```python
from build123d import *

# Parameters (mm, degrees)
F1_DEPTH = 4.5


with BuildPart() as f1:
    # F0 (on Top) → F1 (new body)
    with BuildSketch(Plane.XY):
        with BuildLine():
            Line((-6.747654, 8.625), (3.625, 8.625))
            ThreePointArc((3.625, 8.625), (7.160534, 7.160534), (8.625, 3.625))
            Line((8.625, 3.625), (8.625, -3.625))
            ThreePointArc((8.625, -3.625), (7.160534, -7.160534), (3.625, -8.625))
            Line((3.625, -8.625), (-6.747654, -8.625))
            ThreePointArc((-6.747654, -8.625), (-8.505197, -8.944076), (-10.038423, -9.860582))
            Line((-10.038423, -9.860582), (-12.049675, -11.618772))
            ThreePointArc((-12.049675, -11.618772), (1.752407, -16.64691), (14.204929, -8.854971))
            ThreePointArc((14.204929, -8.854971), (16.021618, -7.128207), (18.44802, -6.5))
            Line((18.44802, -6.5), (43.625, -6.5))
            ThreePointArc((43.625, -6.5), (47.160534, -5.035534), (48.625, -1.5))
            Line((48.625, -1.5), (48.625, 1.5))
            ThreePointArc((48.625, 1.5), (47.160534, 5.035534), (43.625, 6.5))
            Line((43.625, 6.5), (18.44802, 6.5))
            ThreePointArc((18.44802, 6.5), (16.021618, 7.128207), (14.204929, 8.854971))
            ThreePointArc((14.204929, 8.854971), (1.752407, 16.64691), (-12.049675, 11.618772))
            Line((-12.049675, 11.618772), (-10.038423, 9.860582))
            ThreePointArc((-10.038423, 9.860582), (-8.505197, 8.944076), (-6.747654, 8.625))
        make_face()
    extrude(amount=F1_DEPTH)


solid = f1.part
```
Here's how the part is built. I have some questions about the finished solid (model axes, mm). A direction names the side the tool comes from. Round coordinates to 2 decimals unless told otherwise and drop trailing zeros. Order: outer loops, then holes, each group sorted by start corner. A loop starts at its lowest first (then second) coordinate and runs counter-clockwise, first axis right, second up. Notation, with made-up numbers: M -23.75,-32 L 23.25,-32 A21 ccw 23.25,-7 Z; hole C 75.5,23 d2. An arc over 180 degrees is marked long. Use CSV: the item, a comma, the result in double quotes.
1) I want a section at A-A (x = 0). List the corners of the cut face in (y, z) for me (3 decimals), then the cut area to 3 significant figures.
Taken from the geometry:
outline,"M -16.739,0 L -8.625,0 L -8.625,4.5 L -16.739,4.5 Z; M 8.625,0 L 16.739,0 L 16.739,4.5 L 8.625,4.5 Z"
area,"73.0 mm^2"
2) If we mould it in two halves opening along Y, with no side actions, what happens to faces 1 (the cylindrical face through (47.121, -5.074, 2.218)), 2 (the flat face through (-1, -8.625, 2)), 3 (the cylindrical face through (47.199, 4.996, 2.218))? For each: pulls with the +Y half, pulls with the -Y half, needs draft (parallel to the pull), parting line crosses it, or undercut.
Taken from the geometry:
face 1,"pulls with the -Y half"
face 2,"undercut"
face 3,"pulls with the +Y half"
3) I want a section at B-B (z = 2.2). List the corners of the cut face in (x, y) for me (3 decimals), then the cut area to 3 significant figures.
Taken from the geometry:
outline,"M -12.05,-11.619 A16.739 ccw 14.205,-8.855 A5 cw 18.448,-6.5 L 43.625,-6.5 A5 ccw 48.625,-1.5 L 48.625,1.5 A5 ccw 43.625,6.5 L 18.448,6.5 A5 cw 14.205,8.855 A16.739 ccw -12.05,11.619 L -10.038,9.861 A5 ccw -6.748,8.625 L 3.625,8.625 A5 cw 8.625,3.625 L 8.625,-3.625 A5 cw 3.625,-8.625 L -6.748,-8.625 A5 ccw -10.038,-9.861 Z"
area,"861 mm^2"
4) I'm going to push flat-ended pins straight in: P1, Ø2, axis at y = -1.5, z = 3.5, coming from the -X side (3 decimals); P2, Ø2, axis at x = 37.5, z = 1.5, coming from the +Y side; P3, Ø2, axis at x = 16.5, z = 1, coming from the +Y side. Where does each tip first touch, or does it pass through?
Taken from the geometry:
P1,"x = 8.625"
P2,"y = 6.5"
P3,"y = 7.46"
5) I need wall thicknesses on line 1 along X through (y, z) = (1, 3.6) (3 decimals); line 2 along Y through (x, z) = (31, 1.7); line 3 along Y through (x, z) = (3, 2.4) (3 decimals). Which ranges of each line are inside material? Lowest first, please. Write a range as [from, to].
Taken from the geometry:
line 1,"[8.625, 48.625]"
line 2,"[-6.5, 6.5]"
line 3,"[-16.468, -8.625], [8.625, 16.468]"
6) I want a section at D-D (x = 30). List the corners of the cut face in (y, z) for me, then the cut area to 3 significant figures.
Taken from the geometry:
outline,"M -6.5,0 L 6.5,0 L 6.5,4.5 L -6.5,4.5 Z"
area,"58.5 mm^2"
7) I want a section at C-C (y = -8). List the corners of the cut face in (x, z) for me.
Taken from the geometry:
outline,"M 6.05,0 L 14.88,0 L 14.88,4.5 L 6.05,4.5 Z"
8) On a 3-axis mill with a long thin cutter (end or side, diameter ignored), from which of +Z, -Z, +X, -X, +Y, -Y can I reach the whole of each face in a straight line? I mean faces 4 (the flat face through (31, 6.5, 2)), 5 (the flat face through (18, 0, 0)), 6 (the cylindrical face through (7.12, 7.2, 2.22)), 7 (the flat face through (31, -6.5, 2)). Say none if no direction works.
Taken from the geometry:
face 4,"+Z, -Z, +X, +Y"
face 5,"-Z, +X, -X, +Y, -Y"
face 6,"+Z, -Z, -X"
face 7,"+Z, -Z, +X, -Y"
